from build123d import *

# Parameters (mm, degrees)
F2_R            = 60
F3_DEPTH        = 12
F4_R            = 6
F5_DEPTH        = 12.001
F5_COPIES_COUNT = 6


# Not quite as in the source:
# - a pattern or mirror of a feature is missing from the dataset's text; its kind, count and spacing are read off the source's solid


with BuildPart() as f3:
    # F2 (on Top) → F3 (new body)
    with BuildSketch(Plane.XY):
        Circle(F2_R)
    extrude(amount=F3_DEPTH)

    # F4 (on face) → F5 (cut, through all)
    with BuildSketch(Plane.XY.offset(12)):
        with Locations((0, 40)):
            Circle(F4_R)
    f5 = extrude(amount=-F5_DEPTH, mode=Mode.SUBTRACT)

    # F5_copies: F5 ×6 about axis
    f5_copies_axis = Axis((0, 0, 0), (0, 0, 1))
    for i in range(1, F5_COPIES_COUNT):
        add(f5.rotate(f5_copies_axis, i * 360 / F5_COPIES_COUNT), mode=Mode.SUBTRACT)


solid = f3.part
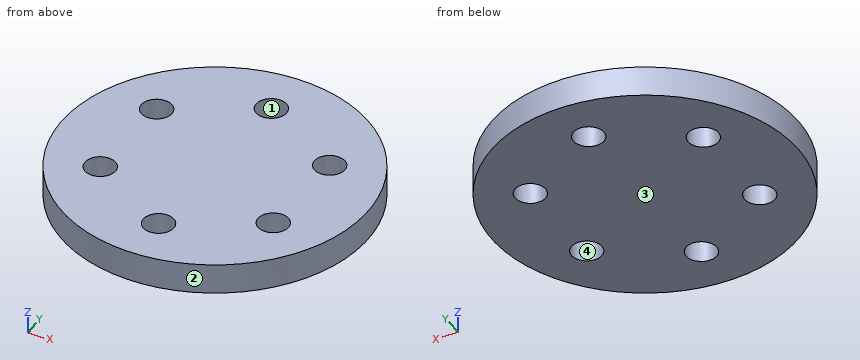
Here's how the part is built. I have some questions about the finished solid (model axes, mm). Face numbers are marked on the shaded views. Give positions to 0.01 mm unless a question says otherwise; leave off trailing zeros. Loops run counter-clockwise (first coordinate to the right, second up) from the corner with the lowest first, then second, coordinate; pieces in that order, holes last. Notation, with made-up numbers: (-39.75, 3) -> (-23.75, 3) arc R27 cw to (-23.75, 30) -> close; hole circle Ø5 at (75, -10.75). An arc over 180 degrees is marked (long way). Answer as a JSON object with one key per item and string values. Group by question number.
Item 1: Imagine slicing it at A-A on x = 0. Write out the boundary of the cut face in (y, z), then the cut area to 3 significant figures.
Item 2: Thinking about a two-plate mould opening in Y: for the marked faces 1, 2, 3 and 4, which applies, pulls with the +Y half, pulls with the -Y half, needs draft (parallel to the pull), parting line crosses it, or undercut?
Item 3: Imagine slicing it at D-D on x = 51.5. Write out the boundary of the cut face in (y, z), then the cut area to 3 significant figures.
Item 4: Imagine slicing it at C-C on y = -40. Write out the boundary of the cut face in (x, z).
Item 5: Will these pins go through, and if not, where does the flat tip stop? pin 1 (15.5 mm diameter, centred on x = 0, y = 40, fed in from -Z); pin 2 (5 mm diameter, centred on x = -7.5, z = 7, fed in from +Y); pin 3 (11 mm diameter, centred on x = 34.64, y = 20, fed in from -Z); pin 4 (1.5 mm diameter, centred on y = -16.5, z = 10.5, fed in from -X).
Item 6: I need wall thicknesses on L1, parallel to Y at x = 0, z = 7; L2, parallel to X at y = -22.5, z = 1.5; L3, parallel to Y at x = -1, z = 8.5. Which ranges of each line are inside material? Lowest first, please.
Item 7: Imagine slicing it at B-B on y = -20. Write out the boundary of the cut face in (x, z).
Answer list:
{
 "1": {"outline": "(-60, 0) -> (-46, 0) -> (-46, 12) -> (-60, 12) -> close; (-34, 0) -> (34, 0) -> (34, 12) -> (-34, 12) -> close; (46, 0) -> (60, 0) -> (60, 12) -> (46, 12) -> close", "area": "1,150 mm2"},
 "2": {"face 1": "undercut", "face 2": "parting line crosses it", "face 3": "needs draft", "face 4": "undercut"},
 "3": {"outline": "(-30.79, 0) -> (30.79, 0) -> (30.79, 12) -> (-30.79, 12) -> close", "area": "739 mm2"},
 "4": {"outline": "(-44.72, 0) -> (-6, 0) -> (-6, 12) -> (-44.72, 12) -> close; (6, 0) -> (44.72, 0) -> (44.72, 12) -> (6, 12) -> close"},
 "5": {"pin 1": "stops at z = 0", "pin 2": "stops at y = 59.79", "pin 3": "passes through", "pin 4": "stops at x = -57.9"},
 "6": {"L1": "y = -60 to -46, -34 to 34, 46 to 60", "L2": "x = -55.62 to -40.1, -29.19 to 29.19, 40.1 to 55.62", "L3": "y = -59.99 to -45.92, -34.08 to 34.08, 45.92 to 59.99"},
 "7": {"outline": "(-56.57, 0) -> (-40.64, 0) -> (-40.64, 12) -> (-56.57, 12) -> close; (-28.64, 0) -> (28.64, 0) -> (28.64, 12) -> (-28.64, 12) -> close; (40.64, 0) -> (56.57, 0) -> (56.57, 12) -> (40.64, 12) -> close"}
}
